Autodesk Inventor part; units mm, degrees
ref_plane "YZ Plane" through (0, 0, 0) normal (1, 0, 0) x (0, 1, 0)
ref_plane "XZ Plane" through (0, 0, 0) normal (0, 1, 0) x (-1, 0, 0)
ref_plane "XY Plane" through (0, 0, 0) normal (0, 0, 1) x (1, 0, 0)
sketch "Sketch1" plane through (0, 0, 0) normal (0, 0, 1) x (1, 0, 0)
  line L0 (0, 8) -> (59.5, 8)
  line L1 (59.5, 8) -> (59.5, -32)
  line L2 (59.5, -32) -> (0, -32)
  line L3 (0, -32) -> (0, 8)
  line L4 (0, 0) -> (0, 3) construction
  line L5 (59.5, 0) -> (59.5, 3) construction
  line L6 (0, 3) -> (16.75, 3) construction
  line L7 (15.75, -25) -> (7.75, -25)
  line L8 (15.75, -25) -> (15.75, -22)
  line L9 (7.75, -22) -> (15.75, -22)
  line L10 (7.75, -25) -> (7.75, -22)
  line L11 (33.75, -25) -> (25.75, -25)
  line L12 (33.75, -25) -> (33.75, -22)
  line L13 (25.75, -22) -> (33.75, -22)
  line L14 (25.75, -25) -> (25.75, -22)
  line L15 (51.75, -25) -> (43.75, -25)
  line L16 (51.75, -25) -> (51.75, -22)
  line L17 (43.75, -22) -> (51.75, -22)
  line L18 (43.75, -25) -> (43.75, -22)
  line L19 (16.75, -15) -> (24.75, -15)
  line L20 (24.75, -15) -> (24.75, -12)
  line L21 (16.75, -12) -> (24.75, -12)
  line L22 (16.75, -15) -> (16.75, -12)
  line L23 (34.75, -15) -> (42.75, -15)
  line L24 (42.75, -15) -> (42.75, -12)
  line L25 (34.75, -12) -> (42.75, -12)
  line L26 (34.75, -15) -> (34.75, -12)
  line L27 (16.75, 0) -> (24.75, 0)
  line L28 (24.75, 0) -> (24.75, 3)
  line L29 (16.75, 3) -> (24.75, 3)
  line L30 (16.75, 0) -> (16.75, 3)
  line L31 (34.75, 0) -> (42.75, 0)
  line L32 (42.75, 0) -> (42.75, 3)
  line L33 (34.75, 3) -> (42.75, 3)
  line L34 (34.75, 0) -> (34.75, 3)
  dimension "d0" = 40
  dimension "d1" = 5
extrude "Extrusion1" add sketch "Sketch1" along normal blind 3
properties part number "Side" material "Polycarbonate, Clear"
Check sheet for the modelled part. Datum: model origin and axes. Units: mm. A direction names the side the tool comes from. Coordinates: 2 decimals unless noted, no trailing zeros. Loops run counter-clockwise (first coordinate to the right, second up) from the corner with the lowest first, then second, coordinate; pieces in that order, holes last.
1) Gauge pin test, flat end, axial feed: pin 1 (8 mm diameter, centred on x = 30.5, y = 1, fed in from -Z). Record the tip position at first contact, or that the pin passes through.
2) Sectioned sample at A-A (x = 45.5). Record the boundary of the cut face in (y, z), and give its area (3 significant figures).
3) Material ranges on probe 1 along X at (y, z) = (-23, 1.95); probe 2 along X at (y, z) = (1, 0.5); probe 3 along Y at (x, z) = (40, 1.9), recorded low to high.
4) Sectioned sample at C-C (x = 37.5). Record the boundary of the cut face in (y, z), and give its area (3 significant figures).
5) Access from +Z, -Z, +X, -X, +Y, -Y to the whole of each face (thin tool, end or side, straight path). Record for faces 1 (the face through (29, -12, 0)), 2 (the face through (43.75, -24, 1)).
6) Release check for a two-part mould opening along Y. For faces 3 (the face through (34.75, -14, 1)), 4 (the face through (39, -12, 1)), 5 (the face through (59.5, -12, 1)) record: released by +Y, released by -Y, zero draft, split by the parting line, or undercut.
7) Sectioned sample at B-B (z = 0.55). Count the separate pieces of the cut face and the enclosed holes in it, and give its area (3 significant figures).
Check sheet entries:
1. pin 1: stops at z = 0
2. outline: (-32, 0) - (-25, 0) - (-25, 3) - (-32, 3) - close; (-22, 0) - (8, 0) - (8, 3) - (-22, 3) - close
2. area: 111 mm2
3. probe 1: x = 0 to 7.75, 15.75 to 25.75, 33.75 to 43.75, 51.75 to 59.5
3. probe 2: x = 0 to 16.75, 24.75 to 34.75, 42.75 to 59.5
3. probe 3: y = -32 to -15, -12 to 0, 3 to 8
4. outline: (-32, 0) - (-15, 0) - (-15, 3) - (-32, 3) - close; (-12, 0) - (0, 0) - (0, 3) - (-12, 3) - close; (3, 0) - (8, 0) - (8, 3) - (3, 3) - close
4. area: 102 mm2
5. face 1: -Z, +X, -X, +Y, -Y
5. face 2: +Z, -Z
6. face 3: undercut
6. face 4: undercut
6. face 5: zero draft
7. separate pieces: 1
7. enclosed holes: 7
7. area: 2,210 mm2
